```python
from build123d import *

# Parameters (mm, degrees)
F1_DEPTH  = 40
F2_R      = 45.5
F3_DEPTH  = 40.001
F4_W      = 20
F4_H      = 25.6125017601
F5_DEPTH  = 40.001
F6_R      = 4.5
F7_DEPTH  = 180.001
F8_R      = 5
F9_DEPTH  = 25.001
F10_R     = 9
F10_R_2   = 5
F11_DEPTH = 9
F12_R     = 5


# Not quite as in the source:
# - a pattern or mirror of a feature is missing from the dataset's text; its kind, count and spacing are read off the source's solid


with BuildPart() as f1:
    # F0 (on Top) → F1 (new body)
    with BuildSketch(Plane.XY):
        Polygon((-105, 25), (-105, 0), (105, 0), (105, 25), (75, 25), (75, 150), (-75, 150), (-75, 25), align=None)
    extrude(amount=F1_DEPTH)

    # F2 (on face) → F3 (cut, through all)
    with BuildSketch(Plane.XY.offset(40)):
        with Locations((0, 80)):
            Circle(F2_R)
    extrude(amount=-F3_DEPTH, mode=Mode.SUBTRACT)

    # F4 (on face) → F5 (cut, through all)
    with BuildSketch(Plane.XY.offset(40)):
        with Locations((0, 137.19374912)):
            Rectangle(F4_W, F4_H)
    extrude(amount=-F5_DEPTH, mode=Mode.SUBTRACT)

    # F6 (on face) → F7 (cut, through all)
    with BuildSketch(Plane.YZ.offset(75)):
        with Locations((135, 20)):
            Circle(F6_R)
    extrude(amount=-F7_DEPTH, mode=Mode.SUBTRACT)

    # F8 (on face) → F9 (cut, through all)
    with BuildSketch(Plane(origin=(0, 25, 0), x_dir=(-1, 0, 0), z_dir=(0, 1, 0))):
        with Locations((90, 20)):
            Circle(F8_R)
    f9 = extrude(amount=-F9_DEPTH, mode=Mode.SUBTRACT)

    # F9_copies: F9 across plane
    add(f9.mirror(Plane(origin=(0, 0, 0), x_dir=(0, 0, 1), z_dir=(1, 0, 0))), mode=Mode.SUBTRACT)

    # F10 (on face) → F11 (cut)
    with BuildSketch(Plane.XZ):
        with Locations((-90, 20)):
            Circle(F10_R)
        with Locations((-90, 20)):
            Circle(F10_R_2, mode=Mode.SUBTRACT)
    f11 = extrude(amount=-F11_DEPTH, mode=Mode.SUBTRACT)

    # F11_copies: F11 across plane
    add(f11.mirror(Plane(origin=(0, 0, 0), x_dir=(0, 0, 1), z_dir=(1, 0, 0))), mode=Mode.SUBTRACT)

    # F12
    f12_edges = [f1.edges().sort_by_distance(p)[0] for p in [
        (-75, 25, 20),
        (75, 25, 20),
    ]]
    fillet(f12_edges, radius=F12_R)


solid = f1.part
```
CAD build for the part. Positions are in the model's coordinates, mm. A direction names the side the tool comes from. Round coordinates to 2 decimals unless told otherwise and drop trailing zeros. Order: outer loops, then holes, each group sorted by start corner. A loop starts at its lowest first (then second) coordinate and runs counter-clockwise, first axis right, second up. Notation, with made-up numbers: (-36.5, 20.5) -> (-29.5, 20.5) arc R26 cw to (-29.5, 37.5) -> close; hole circle Ø9 at (-25, 68.25). An arc over 180 degrees is marked (long way). Write item = value, one per line.
(1) Cut at C-C (y = 80). Write the cut outline in (x, z).
Answers follow:
outline = (-75, 0) -> (-45.5, 0) -> (-45.5, 40) -> (-75, 40) -> close; (45.5, 0) -> (75, 0) -> (75, 40) -> (45.5, 40) -> close
(2) Cut at A-A (y = 135). Write the cut outline in (x, z), plus the area to 3 significant figures.
Answers follow:
outline = (-75, 0) -> (-10, 0) -> (-10, 15.5) -> (-75, 15.5) -> close; (-75, 24.5) -> (-10, 24.5) -> (-10, 40) -> (-75, 40) -> close; (10, 0) -> (75, 0) -> (75, 15.5) -> (10, 15.5) -> close; (10, 24.5) -> (75, 24.5) -> (75, 40) -> (10, 40) -> close
area = 4,030 mm²
(3) Flat gauge pins, fed straight in: P1, Ø7.5, axis at x = -95, z = 26, coming from the +Y side; P2, Ø1, axis at y = 95.5, z = 32.5, coming from the +X side; P3, Ø3, axis at y = 75, z = 11.5, coming from the -X side. Where does each tip first touch, or does it go through?
Answers follow:
P1 = 25
P2 = 75
P3 = -75
(4) Pull direction X, two halves, no side cores. Call faces 1 (the flat face through (-10, 140, 20)), 2 (the flat face through (43, 150, 20)), 3 (the flat face through (-75, 91, 20)): +X half, -X half, draft (parallel to the pull), parting line (faces both ways), or undercut.
Answers follow:
face_1 = undercut
face_2 = draft
face_3 = -X half
(5) 3-axis set-ups, long thin cutter, end or side, ignore diameter. For faces 4 (the flat face through (-86, 9, 16)), 5 (the flat face through (-92, 25, 15)), 6 (the flat face through (95.5, 25, 19.7)): which of +Z, -Z, +X, -X, +Y, -Y reach the whole face in a straight line?
Answers follow:
face_4 = -Y
face_5 = +Z, -Z, -X, +Y
face_6 = +Z, -Z, +X, +Y
(6) Cut at B-B (x = 90). Write the cut outline in (y, z), plus the area to 3 significant figures.
Answers follow:
outline = (0, 0) -> (25, 0) -> (25, 15) -> (9, 15) -> (9, 11) -> (0, 11) -> close; (0, 29) -> (9, 29) -> (9, 25) -> (25, 25) -> (25, 40) -> (0, 40) -> close
area = 678 mm²
(7) Drill centre lines: L1, parallel to X at y = 14, z = 20; L2, parallel to X at y = 11, z = 19; L3, parallel to Z at x = -90, y = 5. Where is each one in solid material? Low to high.
Answers follow:
L1 = -105 to -95, -85 to 85, 95 to 105
L2 = -105 to -94.9, -85.1 to 85.1, 94.9 to 105
L3 = 0 to 11, 29 to 40
(8) Cut at D-D (x = -24). Write the cut outline in (y, z), plus the area to 3 significant figures.
Answers follow:
outline = (0, 0) -> (41.34, 0) -> (41.34, 40) -> (0, 40) -> close; (118.66, 0) -> (150, 0) -> (150, 40) -> (118.66, 40) -> close; hole circle Ø9 at (135, 20)
area = 2,840 mm²
